Part model, mm, in its own coordinate system. Face numbers are marked on the shaded views. Round coordinates to 2 decimals unless told otherwise and drop trailing zeros. Loops run counter-clockwise (first coordinate to the right, second up) from the corner with the lowest first, then second, coordinate; pieces in that order, holes last. Notation, with made-up numbers: (82.25, 3.5) -> (139.25, 3.5) arc R17 cw to (139.25, 29.5) -> close; hole circle Ø4 at (40.25, 51.25). An arc over 180 degrees is marked (long way). Answer as CSV lines item,"result".
Autodesk Fusion 360 part; units mm, degrees
sketch "Sketch1" plane through (0, 0, 0) normal (0, 0, 1) x (1, 0, 0)
  circle A0 centre (0, 0) radius 8.15
  circle A1 centre (0, 0) radius 9.15 construction
  circle A2 centre (0, 0) radius 10.15 construction
  line L0 (-5.8601, 10.15) -> (-11.7202, 0)
  line L1 (-11.7202, 0) -> (-5.8601, -10.15)
  line L2 (-5.8601, -10.15) -> (5.8601, -10.15)
  line L3 (5.8601, -10.15) -> (11.7202, 0)
  line L4 (11.7202, 0) -> (5.8601, 10.15)
  line L5 (5.8601, 10.15) -> (-5.8601, 10.15)
  dimension "d1" = 16.3
  dimension "d2" = 1
  dimension "d3" = 2
extrude "Extrude1" add sketch "Sketch1" along normal blind 10
fillet "Fillet1" radius 1 6 edges at (-8.7902, 5.075, 10) (-8.7902, -5.075, 10) (0, -10.15, 10) (8.7902, -5.075, 10) (8.7902, 5.075, 10) (0, 10.15, 10)
fillet "Fillet2" radius 1 6 edges at (0, 10.15, 0) (8.7902, 5.075, 0) (8.7902, -5.075, 0) (0, -10.15, 0) (-8.7902, -5.075, 0) (-8.7902, 5.075, 0)
thread "Thread1"
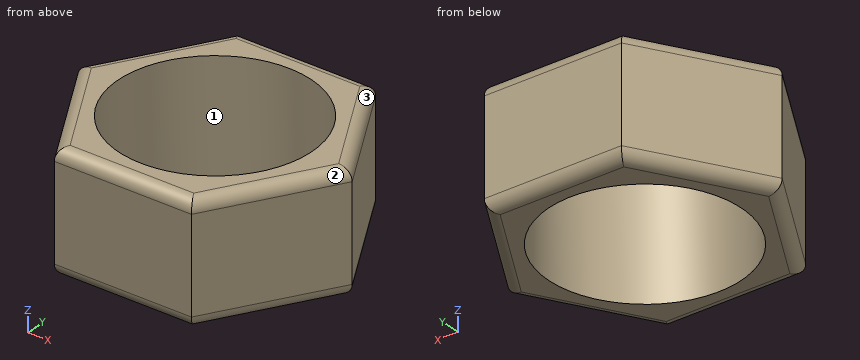
Q1. Saw through at C-C, the plane x = 0. Write the cut outline in (y, z).
Geometry results:
outline,"(-10.15, 1) arc R1 ccw to (-9.15, 0) -> (-8.15, 0) -> (-8.15, 10) -> (-9.15, 10) arc R1 ccw to (-10.15, 9) -> close; (8.15, 0) -> (9.15, 0) arc R1 ccw to (10.15, 1) -> (10.15, 9) arc R1 ccw to (9.15, 10) -> (8.15, 10) -> close"
Q2. Drop flat-ended pins along their axis: P1, Ø2, axis at y = 7, z = 7.5, coming from the -X side; P2, Ø6, axis at x = 1.5, y = 7.5, coming from the +Z side; P3, Ø2, axis at y = 3.5, z = 1, coming from the -X side. Give the stop position or say it passes through.
Geometry results:
P1,"x = -8.26"
P2,"z = 10"
P3,"x = -10.28"
Q3. Saw through at B-B, the plane z = 5. Write the cut outline in (x, y).
Geometry results:
outline,"(-11.72, 0) -> (-5.86, -10.15) -> (5.86, -10.15) -> (11.72, 0) -> (5.86, 10.15) -> (-5.86, 10.15) -> close; hole circle Ø16.3 at (0, 0)"
Q4. Two-plate mould, pull along Y, no slides. Class the marked faces 1, 2 and 3: pulls with the +Y half, pulls with the -Y half, needs draft (parallel to the pull), parting line crosses it, or undercut.
Geometry results:
face 1,"undercut"
face 2,"pulls with the -Y half"
face 3,"pulls with the +Y half"
Q5. Saw through at A-A, the plane x = 5. Write the cut outline in (y, z).
Geometry results:
outline,"(-10.15, 1) arc R1 ccw to (-9.15, 0) -> (-6.44, 0) -> (-6.44, 10) -> (-9.15, 10) arc R1 ccw to (-10.15, 9) -> close; (6.44, 0) -> (9.15, 0) arc R1 ccw to (10.15, 1) -> (10.15, 9) arc R1 ccw to (9.15, 10) -> (6.44, 10) -> close"
Q6. Drill centre lines: line 1 along Y through (x, z) = (-0.25, 3.75); line 2 along Y through (x, z) = (-3.25, 2.5); line 3 along X through (y, z) = (6.25, 4.5). Where is each one in solid material? Low to high.
Geometry results:
line 1,"-10.15 to -8.15, 8.15 to 10.15"
line 2,"-10.15 to -7.47, 7.47 to 10.15"
line 3,"-8.11 to -5.23, 5.23 to 8.11"
